Geometry: final body of the model. Coordinates: model frame, mm. Face numbers are marked on the shaded views. A direction names the side the tool comes from. Coordinates: 2 decimals unless noted, no trailing zeros. Write each loop counter-clockwise with the first axis right and the second up, starting at its lowest first coordinate (ties: lowest second). Pieces come first, ordered by that corner, then holes. Notation, with made-up numbers: (47, -21.75) - (76, -21.75) arc R11 cw to (76, -12.75) - close; hole circle Ø6 at (72, 58.25). An arc over 180 degrees is marked (long way). Answer as a JSON object with one key per item and string values. Group by question number.
Item 1: Section A-A on z = 17.25. Return loops of the section in (x, y), and give its area (3 significant figures).
Item 2: Mould query, pull axis Y, two halves, no side actions, for the marked faces 3, 4, 5 and 6. Classes: pulls with the +Y half, pulls with the -Y half, needs draft (parallel to the pull), parting line crosses it, or undercut.
Item 3: Set-up query: the marked faces 1 and 2. Return all of +Z, -Z, +X, -X, +Y, -Y with unobstructed straight access to the full face (end or side cutting, diameter ignored); none if empty.
Item 4: Section C-C on y = -15.5. Return loops of the section in (x, z) (3 decimals), and give its area (3 significant figures).
Item 5: Section D-D on x = -44.5. Return loops of the section in (y, z) (3 decimals).
Item 6: Section B-B on x = 18. Return loops of the section in (y, z) (3 decimals), and give its area (3 significant figures).
Item 7: First-contact query: pin 1 Ø4 at (y, z) = (6, 16) entering from -X; pin 2 Ø19.5 at (x, y) = (-12, -9) entering from +Z (3 decimals); pin 3 Ø4 at (y, z) = (8.5, 21) entering from -X; pin 4 Ø10 at (x, y) = (44.04, -10.19) entering from +Z. Flat tips, straight axial feed; report the tip coordinate or a pass-through.
Item 8: Line query: line 1 along Y through (x, z) = (-14, 23.75); line 2 along X through (y, z) = (-14.5, 8.25); line 3 along X through (y, z) = (-12, 2.75). Output: solid intervals per line, ascending. Write a range as from..to.
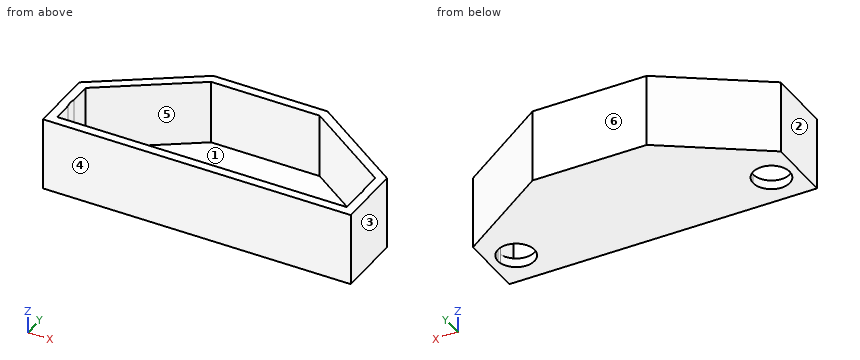
```python
from build123d import *

# Parameters (mm, degrees)
F1_DEPTH = 25.4
F2_DEPTH = 3.175


with BuildPart() as f1:
    # F0 (on Top) → F1 (new body)
    with BuildSketch(Plane.XY):
        Polygon((-53.3932372928, -22.7622538805), (53.3932372928, -22.7622538805), (53.3932372928, 0), (20.1804766856, 22.7622538805), (-19.4478705525, 22.7622538805), (-53.3932372928, 0), align=None)
        with BuildLine():
            Line((50.2182372928, -11.6402664429), (50.2182372928, -19.5872538805))
            Line((50.2182372928, -19.5872538805), (-50.2182372928, -19.5872538805))
            Line((-50.2182372928, -19.5872538805), (-50.2182372928, -12.7441667186))
            ThreePointArc((-50.2182372928, -12.7441667186), (-50.4958895802, -10.8869932592), (-50.2182372928, -9.0298197998))
            Line((-50.2182372928, -9.0298197998), (-50.2182372928, -1.6937240379))
            Line((-50.2182372928, -1.6937240379), (-18.4818985354, 19.5872538805))
            Line((-18.4818985354, 19.5872538805), (19.1969012537, 19.5872538805))
            Line((19.1969012537, 19.5872538805), (50.2182372928, -1.6731145359))
            Line((50.2182372928, -1.6731145359), (50.2182372928, -8.7388372773))
            ThreePointArc((50.2182372928, -8.7388372773), (50.3440488555, -9.459350693), (50.3861723304, -10.1895518601))
            ThreePointArc((50.3861723304, -10.1895518601), (50.3440488555, -10.9197530272), (50.2182372928, -11.6402664429))
        make_face(mode=Mode.SUBTRACT)
    extrude(amount=F1_DEPTH)

    # F0 (on Top) → F2 (join)
    with BuildSketch(Plane.XY):
        with BuildLine():
            Line((-50.2182372928, -19.5872538805), (50.2182372928, -19.5872538805))
            Line((50.2182372928, -19.5872538805), (50.2182372928, -11.6402664429))
            ThreePointArc((50.2182372928, -11.6402664429), (37.6861723304, -10.1895518601), (50.2182372928, -8.7388372773))
            Line((50.2182372928, -8.7388372773), (50.2182372928, -1.6731145359))
            Line((50.2182372928, -1.6731145359), (19.1969012537, 19.5872538805))
            Line((19.1969012537, 19.5872538805), (-18.4818985354, 19.5872538805))
            Line((-18.4818985354, 19.5872538805), (-50.2182372928, -1.6937240379))
            Line((-50.2182372928, -1.6937240379), (-50.2182372928, -9.0298197998))
            ThreePointArc((-50.2182372928, -9.0298197998), (-43.2069827623, -4.6067899196), (-37.7958895802, -10.8869932592))
            ThreePointArc((-37.7958895802, -10.8869932592), (-43.2069827623, -17.1671965988), (-50.2182372928, -12.7441667186))
            Line((-50.2182372928, -12.7441667186), (-50.2182372928, -19.5872538805))
        make_face()
    extrude(amount=F2_DEPTH)


solid = f1.part
```
Checks:
{
 "1": {"outline": "(-53.39, -22.76) - (53.39, -22.76) - (53.39, 0) - (20.18, 22.76) - (-19.45, 22.76) - (-53.39, 0) - close; hole (-50.22, -19.59) - (50.22, -19.59) - (50.22, -11.64) arc R6.35 ccw to (50.22, -8.74) - (50.22, -1.67) - (19.2, 19.59) - (-18.48, 19.59) - (-50.22, -1.69) - (-50.22, -9.03) arc R6.35 ccw to (-50.22, -12.74) - close", "area": "829 mm^2"},
 "2": {"face 3": "needs draft", "face 4": "pulls with the -Y half", "face 5": "undercut", "face 6": "pulls with the +Y half"},
 "3": {"face 1": "+Z", "face 2": "+Z, -Z, -X, +Y, -Y"},
 "4": {"outline": "(-53.393, 0) - (-48.51, 0) - (-48.51, 3.175) - (-50.218, 3.175) - (-50.218, 25.4) - (-53.393, 25.4) - close; (-39.782, 0) - (40.555, 0) - (40.555, 3.175) - (-39.782, 3.175) - close; (47.518, 0) - (53.393, 0) - (53.393, 25.4) - (50.218, 25.4) - (50.218, 3.175) - (47.518, 3.175) - close", "area": "430 mm^2"},
 "5": {"outline": "(-22.762, 0) - (-17.227, 0) - (-17.227, 3.175) - (-19.587, 3.175) - (-19.587, 25.4) - (-22.762, 25.4) - close; (-4.547, 0) - (5.963, 0) - (5.963, 25.4) - (2.141, 25.4) - (2.141, 3.175) - (-4.547, 3.175) - close"},
 "6": {"outline": "(-22.762, 0) - (22.762, 0) - (22.762, 25.4) - (19.587, 25.4) - (19.587, 3.175) - (-19.587, 3.175) - (-19.587, 25.4) - (-22.762, 25.4) - close", "area": "286 mm^2"},
 "7": {"pin 1": "x = -47.43", "pin 2": "z = 3.175", "pin 3": "x = -43.7", "pin 4": "through"},
 "8": {"line 1": "-22.76..-19.59, 19.59..22.76", "line 2": "-53.39..-50.22, 50.22..53.39", "line 3": "-53.39..-50.4, -37.89..37.95, 50.12..53.39"}
}
